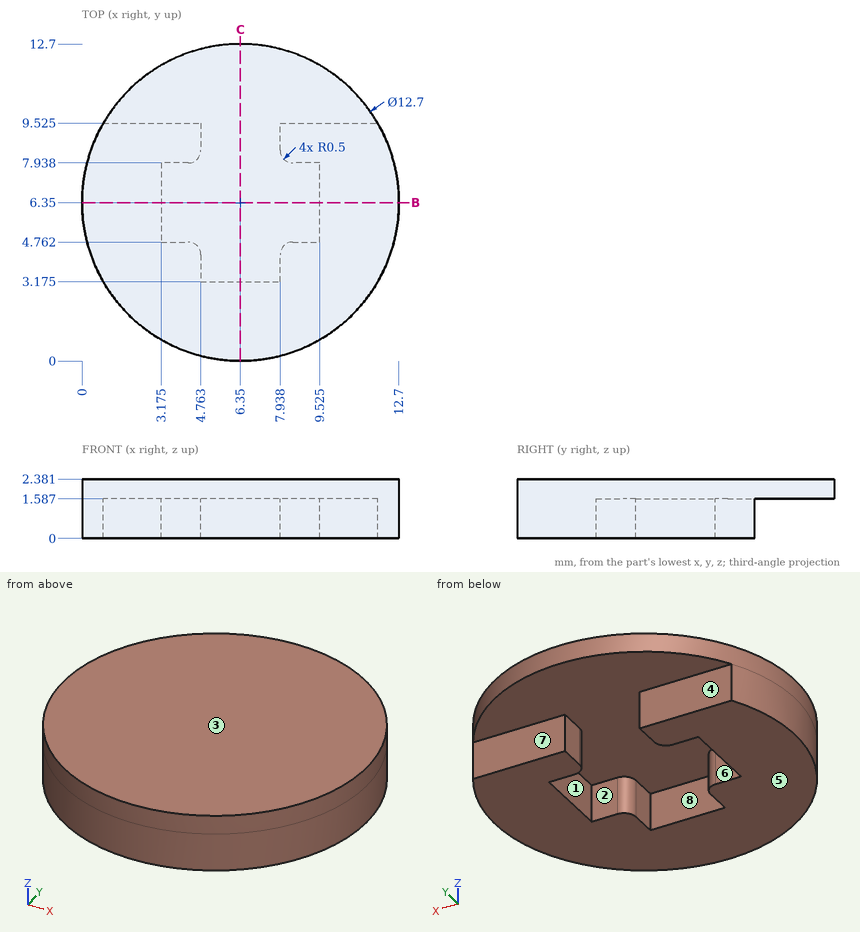
Input: dimensioned drawing with shaded views. Units: mm. Origin: part minimum x, y, z. A direction names the side the tool comes from. Coordinates: 2 decimals unless noted, no trailing zeros. Order: outer loops, then holes, each group sorted by start corner. A loop starts at its lowest first (then second) coordinate and runs counter-clockwise, first axis right, second up. Notation, with made-up numbers: (54, 3) - (100, 3) arc R25 cw to (100, 33) - close; hole circle Ø5 at (61, 39). An arc over 180 degrees is marked (long way). Return JSON: item names as keys, results as strings. Group by question number.
1. Cut plane C-C (x = 6.35). Output: boundary loops of the cut face in (y, z) (1 decimal).
2. Cut plane B-B (y = 6.35). Output: boundary loops of the cut face in (x, z) (1 decimal).
3. Material intervals for line 1 along Y through (x, z) = (4.5, 1.2) (1 decimal); line 2 along Z through (x, y) = (7.5, 12.25); line 3 along X through (y, z) = (4, 0.7), sorted ascending. Write a range as [from, to].
4. Pull-direction query (Y, two-part tool) for the marked faces 1, 2, 3 and 4; classes: pulls with the +Y half, pulls with the -Y half, needs draft (parallel to the pull), parting line crosses it, or undercut.
5. Pin query (flat end, axial travel): pin 1 (0.9 mm diameter, centred on y = 9, z = 0.5, fed in from -X); pin 2 (0.5 mm diameter, centred on y = 7, z = 1, fed in from -X); pin 3 (0.5 mm diameter, centred on x = 4, z = 0.5, fed in from +Y) (1 decimal). Return the tip coordinate at first contact, or that it passes through.
6. Set-up query: the marked faces 5, 6, 7 and 8. Return all of +Z, -Z, +X, -X, +Y, -Y with unobstructed straight access to the full face (end or side cutting, diameter ignored); none if empty.
Resolved:
{
 "1": {"outline": "(0, 0) - (3.2, 0) - (3.2, 1.6) - (12.7, 1.6) - (12.7, 2.4) - (0, 2.4) - close"},
 "2": {"outline": "(0, 0) - (3.2, 0) - (3.2, 1.6) - (9.5, 1.6) - (9.5, 0) - (12.7, 0) - (12.7, 2.4) - (0, 2.4) - close"},
 "3": {"line 1": "y = [0.3, 4.7], [8, 9.5]", "line 2": "z = [1.59, 2.38]", "line 3": "x = [0.45, 4.76], [7.94, 12.25]"},
 "4": {"face 1": "undercut", "face 2": "undercut", "face 3": "needs draft", "face 4": "pulls with the +Y half"},
 "5": {"pin 1": "stops at x = 0.39", "pin 2": "stops at x = 0.01", "pin 3": "stops at y = 9.5"},
 "6": {"face 5": "-Z, +X, -X, +Y, -Y", "face 6": "-Z", "face 7": "-Z, +X, -X, +Y", "face 8": "-Z, +Y"}
}
